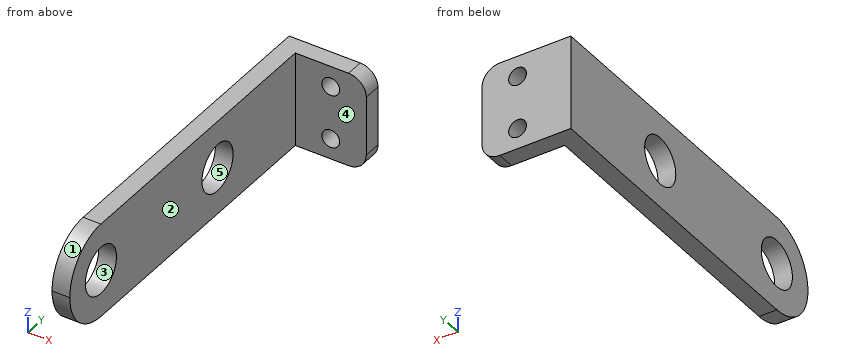
Autodesk Inventor part; units mm, degrees
ref_plane "YZ Plane" through (0, 0, 0) normal (1, 0, 0) x (0, 1, 0)
ref_plane "XZ Plane" through (0, 0, 0) normal (0, 1, 0) x (-1, 0, 0)
ref_plane "XY Plane" through (0, 0, 0) normal (0, 0, 1) x (1, 0, 0)
sketch "Sketch1" plane through (0, 0, 0) normal (0, 0, 1) x (1, 0, 0)
  line L0 (0, 0) -> (0, 61)
  line L1 (3, 0) -> (3, 58)
  line L2 (0, 0) -> (3, 0)
  line L3 (3, 58) -> (15, 58)
  line L4 (0, 61) -> (15, 61)
  line L5 (15, 58) -> (15, 61)
  point P0 (9, 61)
  dimension "d0" = 61
  dimension "d2" = 3
  dimension "d3" = 12
  dimension "d4" = 3
extrude "Extrusion1" add sketch "Sketch1" along normal blind 16
fillet "Fillet1" radius 8 2 edges at (1.5, 0, 16) (1.5, 0, 0)
sketch "Sketch2" plane through (3, 58, 16) normal (1, 0, 0) x (0, 0, -1)
  arc A0 (0, -50) -> (16, -50) centre (8, -50) ccw construction
  line L0 (16, -50) -> (16, 0) construction
  line L1 (16, 0) -> (0, 0) construction
  line L2 (0, -50) -> (0, 0) construction
  line L3 (16, 3) -> (0, 3)
  point P0 (16, -58)
  point P1 (8, -20)
  dimension "d8" = 30
  dimension "d9" = 23
  dimension "d10" = 8
  dimension "d11" = 8
hole "Hole1" at (3, 8, 8) at (3, 38, 8) direction (-1, 0, 0) diameter 8 end through all
sketch "Sketch3" plane through (0, 61, 0) normal (0, 1, 0) x (1, 0, 0)
  line L0 (15, 0) -> (0, 0)
  line L1 (0, 0) -> (0, -16)
  line L2 (15, -16) -> (0, -16)
  line L3 (15, 0) -> (15, -16)
  point P0 (9, -12.5)
  point P1 (9, -3.5)
  point P2 (0, -8)
  dimension "d19" = 9
  dimension "d20" = 9
  dimension "d21" = 4.5
hole "Hole2" at (9, 61, 12.5) at (9, 61, 3.5) direction (0, -1, 0) diameter 3 end through all
fillet "Fillet2" radius 3 2 edges at (15, 59.5, 16) (15, 59.5, 0)
properties part number "HUDSON-1-75"
Input: part model. Units: mm. Frame: model coordinates. Face numbers are marked on the shaded views. A direction names the side the tool comes from. Give positions to 0.01 mm unless a question says otherwise; leave off trailing zeros. Write each loop counter-clockwise with the first axis right and the second up, starting at its lowest first coordinate (ties: lowest second). Pieces come first, ordered by that corner, then holes.
Q1. Pull-direction query (Z, two-part tool) for the marked faces 1, 2 and 3; classes: pulls with the +Z half, pulls with the -Z half, needs draft (parallel to the pull), parting line crosses it, or undercut.
Q2. Section B-B, the plane y = 9.5. Output: boundary loops of the cut face in (x, z).
Q3. Section C-C, the plane z = 6. Output: boundary loops of the cut face in (x, y), plus the area to 3 significant figures.
Q4. Section A-A, the plane x = 9. Output: boundary loops of the cut face in (y, z), plus the area to 3 significant figures.
Q5. Material intervals for probe 1 along Y at (x, z) = (2.35, 8); probe 2 along Z at (x, y) = (9, 59.8); probe 3 along Z at (x, y) = (0.65, 8), sorted ascending.
Q6. Section D-D, the plane y = 31.5. Output: boundary loops of the cut face in (x, z).
Q7. First-contact query: P1, Ø8, axis at y = 48.5, z = 7.5, coming from the +X side; P2, Ø3.5, axis at x = 9, z = 8, coming from the -Y side. Flat tips, straight axial feed; report the tip coordinate or a pass-through.
Q8. Set-up query: the marked faces 4 and 5. Return all of +Z, -Z, +X, -X, +Y, -Y with unobstructed straight access to the full face (end or side cutting, diameter ignored); none if empty.
Filled in:
1. face 1: pulls with the +Z half
1. face 2: needs draft
1. face 3: undercut
2. outline: (0, 0) - (3, 0) - (3, 4.29) - (0, 4.29) - close; (0, 11.71) - (3, 11.71) - (3, 16) - (0, 16) - close
3. outline: (0, 0.25) - (3, 0.25) - (3, 4.54) - (0, 4.54) - close; (0, 11.46) - (3, 11.46) - (3, 34.54) - (0, 34.54) - close; (0, 41.46) - (3, 41.46) - (3, 58) - (15, 58) - (15, 61) - (0, 61) - close
3. area: 177 mm2
4. outline: (58, 0) - (61, 0) - (61, 2) - (58, 2) - close; (58, 5) - (61, 5) - (61, 11) - (58, 11) - close; (58, 14) - (61, 14) - (61, 16) - (58, 16) - close
4. area: 30.0 mm2
5. probe 1: y = 0 to 4, 12 to 34, 42 to 61
5. probe 2: z = 0 to 2, 5 to 11, 14 to 16
5. probe 3: z = 0 to 4, 12 to 16
6. outline: (0, 0) - (3, 0) - (3, 16) - (0, 16) - close
7. P1: stops at x = 3
7. P2: stops at y = 58
8. face 4: +Z, -Z, +X, -Y
8. face 5: +X, -X
